Design review of the part shown in the three views and the two pictorial views. Dimensions are in mm from the part's minimum x, y and z. Round coordinates to 2 decimals unless told otherwise and drop trailing zeros. Loops run counter-clockwise (first coordinate to the right, second up) from the corner with the lowest first, then second, coordinate; pieces in that order, holes last.
1. To check wall thickness, follow line 1 along X through (y, z) = (4, 55); line 2 along Z through (x, y) = (25, 10); line 3 along X through (y, z) = (7, 42.5). State the ranges of each line that lie inside material, in increasing order.
2. Clearance check with a flat-ended pin moving along its axis: pin 1 Ø18 at (x, z) = (25, 50) entering from -Y. State where the tip first meets the part, or that it passes through.
3. Consider section B-B on x = 425. State the section outline as (y, z) points.
4. Consider section A-A on z = 50. State the section outline as (x, y) points, then the cut area to 3 significant figures.
5. Draft analysis for pull direction Y (two halves, no side actions). For the marked faces 1 and 2, state which applies: released by +Y, released by -Y, zero draft, split by the parting line, or undercut.
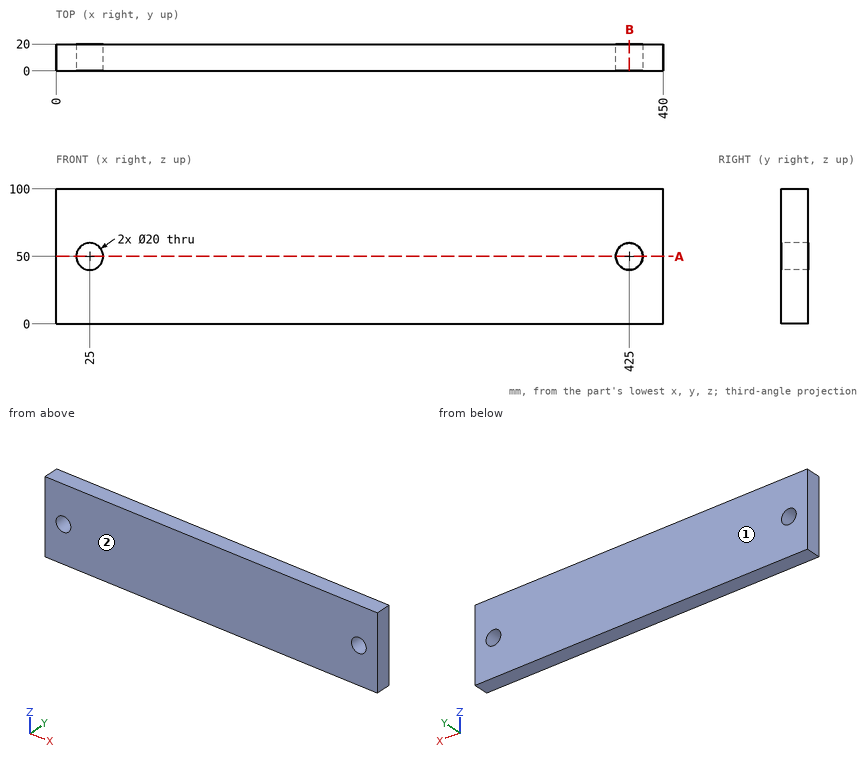
Resolved:
1. line 1: x = 0 to 16.34, 33.66 to 416.34, 433.66 to 450
1. line 2: z = 0 to 40, 60 to 100
1. line 3: x = 0 to 18.39, 31.61 to 418.39, 431.61 to 450
2. pin 1: passes through
3. outline: (0, 0) - (20, 0) - (20, 40) - (0, 40) - close; (0, 60) - (20, 60) - (20, 100) - (0, 100) - close
4. outline: (0, 0) - (15, 0) - (15, 20) - (0, 20) - close; (35, 0) - (415, 0) - (415, 20) - (35, 20) - close; (435, 0) - (450, 0) - (450, 20) - (435, 20) - close
4. area: 8,200 mm2
5. face 1: released by +Y
5. face 2: released by -Y
